from build123d import *

# Parameters (mm, degrees)
F0_R     = 3.3655
F1_DEPTH = 30.0482
F2_R     = 2.6035
F3_DEPTH = 7.747
F5_DEPTH = 7.0358
F7_DEPTH = 5.335


with BuildPart() as f1:
    # F0 (on Right) → F1 (new body)
    with BuildSketch(Plane.YZ):
        Circle(F0_R)
    extrude(amount=-F1_DEPTH)

    # F2 (on face) → F3 (join)
    with BuildSketch(Plane.YZ):
        Circle(F2_R)
    extrude(amount=F3_DEPTH)

    # F4 (on Top) → F5 (join)
    with BuildSketch(Plane.XY):
        with BuildLine():
            Line((-9.4615, 1.9685), (-26.7335, 1.9685))
            ThreePointArc((-26.7335, 1.9685), (-28.702, 0), (-26.7335, -1.9685))
            Line((-26.7335, -1.9685), (-9.4615, -1.9685))
            ThreePointArc((-9.4615, -1.9685), (-7.493, 0), (-9.4615, 1.9685))
        make_face()
    extrude(amount=F5_DEPTH)

    # F6 (on face) → F7 (cut, through all)
    with BuildSketch(Plane.XZ.offset(1.9685)):
        Polygon((-7.493, 7.0358), (-28.702, 7.0358), (-7.493, 6.7818), align=None)
    extrude(amount=-F7_DEPTH, mode=Mode.SUBTRACT)


solid = f1.part
Can you work these out from the model? Positions are in its coordinate system, mm. A direction names the side the tool comes from. Give positions to 0.01 mm unless a question says otherwise; leave off trailing zeros. Loops run counter-clockwise (first coordinate to the right, second up) from the corner with the lowest first, then second, coordinate; pieces in that order, holes last. Notation, with made-up numbers: (19.25, 40.25) -> (34.25, 40.25) arc R17 cw to (34.25, 60.25) -> close; hole circle Ø4 at (77.25, 15). An arc over 180 degrees is marked (long way). Use one line per item in the form item = value.
1) If we section it at C-C (x = 5): Please give me the cut outline in (y, z).
Answers:
outline = circle Ø5.21 at (0, 0)
2) If we section it at D-D (z = 1.75): Please give me the cut outline in (x, y).
Answers:
outline = (-30.05, -2.87) -> (0, -2.87) -> (0, -1.93) -> (7.75, -1.93) -> (7.75, 1.93) -> (0, 1.93) -> (0, 2.87) -> (-30.05, 2.87) -> close
3) I need wall thicknesses on line 1 along X through (y, z) = (0, 3.75); line 2 along X through (y, z) = (1.25, 2.5); line 3 along Y through (x, z) = (-9, -2). Which ranges of each line are inside material? Lowest first, please.
Answers:
line_1 = -28.7 to -7.49
line_2 = -30.05 to 0
line_3 = -2.71 to 2.71
4) If we section it at B-B (y = 0): Please give me the cut outline in (x, z), plus the area to 3 significant figures.
Answers:
outline = (-30.05, -3.37) -> (0, -3.37) -> (0, -2.6) -> (7.75, -2.6) -> (7.75, 2.6) -> (0, 2.6) -> (0, 3.37) -> (-7.49, 3.37) -> (-7.49, 6.78) -> (-28.7, 7.04) -> (-28.7, 3.37) -> (-30.05, 3.37) -> close
area = 318 mm²
5) For faces 1 (the face through (-18, -1.968, 5)), 2 (the face through (-7.493, -0.043, 4.739)), 3 (the face through (-18, 1.968, 5)), 4 (the face through (0, 2, -2)), 5 (the face through (-28.7, 0.04, 4.85)), which set-ups out of +Z, -Z, +X, -X, +Y, -Y let a thin tool reach every point of the face, with its end or its side?
Answers:
face_1 = +Z, +X, -X, -Y
face_2 = +Z, +X
face_3 = +Z, +X, -X, +Y
face_4 = +X
face_5 = +Z, -X
6) Will these pins go through, and if not, where does the flat tip stop? pin 1 (2 mm diameter, centred on x = -15.5, z = 5, fed in from +Y); pin 2 (4 mm diameter, centred on x = 3.5, y = 2.5, fed in from +Z); pin 3 (4.5 mm diameter, centred on x = -17.5, z = 4, fed in from -Y).
Answers:
pin_1 = 1.97
pin_2 = 2.56
pin_3 = -2.87
7) If we section it at A-A (z = 0): Please give me the cut outline in (x, y), plus the area to 3 significant figures.
Answers:
outline = (-30.05, -3.37) -> (0, -3.37) -> (0, -2.6) -> (7.75, -2.6) -> (7.75, 2.6) -> (0, 2.6) -> (0, 3.37) -> (-30.05, 3.37) -> close
area = 243 mm²
